```python
from build123d import *

# Parameters (mm, degrees)
SKETCH1_R           = 5
BOSS_EXTRUDE1_DEPTH = 20
SKETCH2_R           = 4
BOSS_EXTRUDE2_DEPTH = 68
FILLET1_R           = 3.4
CHAMFER1_SIZE       = 11.430052303
CHAMFER1_SIZE_2     = 1
SKETCH3_W           = 5
SKETCH3_H           = 5
CUT_EXTRUDE1_DEPTH  = 8
SKETCH4_W           = 5
SKETCH4_H           = 2.702388579
CUT_EXTRUDE2_DEPTH  = 8
SKETCH5_R           = 0.5
BOSS_EXTRUDE3_DEPTH = 5


with BuildPart() as part:
    # Sketch1 → Boss-Extrude1 (new body)
    with BuildSketch(Plane(origin=(0, 0, 0), x_dir=(1, 0, 0), z_dir=(0, 1, 0))):
        with Locations(Location((0, 0, 0), (0, 0, 270))):
            Circle(SKETCH1_R)
    extrude(amount=BOSS_EXTRUDE1_DEPTH)

    # Sketch2 → Boss-Extrude2 (add)
    with BuildSketch(Plane(origin=(0, 20, 0), x_dir=(1, 0, 0), z_dir=(0, 1, 0))):
        with Locations(Location((0, 0, 0), (0, 0, 270))):
            Circle(SKETCH2_R)
    extrude(amount=BOSS_EXTRUDE2_DEPTH)

    # Fillet1
    fillet1_edges = [part.edges().sort_by_distance(p)[0] for p in [
        (0, 88, -4),
    ]]
    fillet(fillet1_edges, radius=FILLET1_R)

    # Chamfer1
    # the kernel refuses this chamfer: 11.430052303, 1 mm, written as the material it adds along each edge
    with BuildSketch(Plane(origin=(0, 20, 0), x_dir=(0, 0, 1), z_dir=(-1, 0, 0))) as chamfer1_piece_1_section:
        Polygon((4, CHAMFER1_SIZE), (4 + CHAMFER1_SIZE_2, 0), (4, 0), align=None)
    chamfer1_piece_1 = revolve(axis=Axis((0, 20, 0), (0, 1, 0)), mode=Mode.PRIVATE)
    chamfer1_piece_1 = chamfer1_piece_1 & Plane(origin=(0, 25.937398898, 0), x_dir=(0, 0, 1), z_dir=(0, -1, 0)) * Cylinder(5, 46, mode=Mode.PRIVATE)
    add(chamfer1_piece_1)

    # Sketch3 → Cut-Extrude1 (cut)
    with BuildSketch(Plane(origin=(0, 0, 0), x_dir=(-1, 0, 0), z_dir=(0, -1, 0))):
        Rectangle(SKETCH3_W, SKETCH3_H)
    extrude(amount=-CUT_EXTRUDE1_DEPTH, mode=Mode.SUBTRACT)

    # Sketch4 → Cut-Extrude2 (cut)
    with BuildSketch(Plane(origin=(0, 0, 0), x_dir=(-1, 0, 0), z_dir=(0, -1, 0))):
        with Locations((0, 3.851194289)):
            Rectangle(SKETCH4_W, SKETCH4_H)
    extrude(amount=-CUT_EXTRUDE2_DEPTH, mode=Mode.SUBTRACT)

    # Sketch5 → Boss-Extrude3 (add)
    with BuildSketch(Plane.ZY.offset(-2.5)):
        with Locations(Location((0, 5.5, 0), (0, 0, 180))):
            Circle(SKETCH5_R)
    extrude(amount=BOSS_EXTRUDE3_DEPTH)


solid = part.part
```
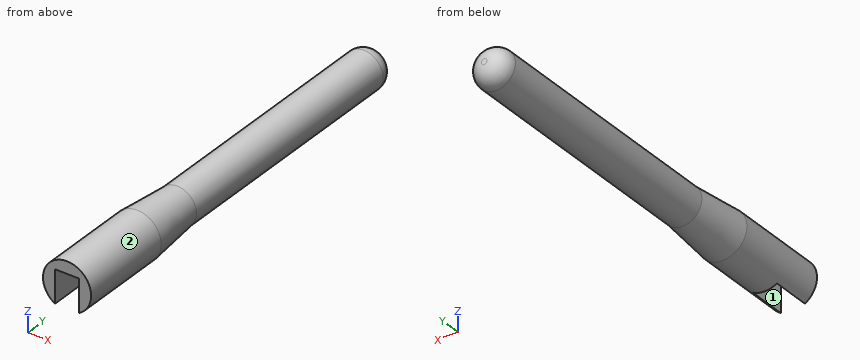
Work out the finished part from the listing and answer in its coordinate system (mm). Face numbers are marked on the shaded views. Coordinates: 2 decimals unless noted, no trailing zeros. Order: outer loops, then holes, each group sorted by start corner. A loop starts at its lowest first (then second) coordinate and runs counter-clockwise, first axis right, second up. Notation, with made-up numbers: M -37.75,2.25 L -31.75,2.25 A23 cw -31.75,36.25 Z; hole C 45,28.25 d8. An arc over 180 degrees is marked long. Use CSV: the item, a comma, the result in double quotes.
1) Determine the mould class of the marked faces 1 and 2 for opening direction X: released by +X, released by -X, zero draft, split by the parting line, or undercut.
Worked out:
face 1,"undercut"
face 2,"split by the parting line"
2) Flat-ended cylindrical pins translate along their axes: pin 1 Ø3.5 at (y, z) = (4, -2.5) entering from +X; pin 2 Ø3 at (y, z) = (45.5, -1.5) entering from -X; pin 3 Ø1.5 at (x, y) = (0.5, 4) entering from -Z. Find the tip coordinate at first contact, or state that the pin passes through.
Worked out:
pin 1,"stops at x = 4.94"
pin 2,"stops at x = -4"
pin 3,"stops at z = 2.5"
3) Section B-B on y = 10 is taken. Write down the section's boundary in (x, z).
Worked out:
outline,"C 0,0 d10"
4) Section A-A on y = 66.5 is taken. Write down the section's boundary in (x, z), plus the area to 3 significant figures.
Worked out:
outline,"C 0,0 d8"
area,"50.3 mm^2"
5) Consider line 1 (Z direction, x = -2.75, y = 21.5); line 2 (Y direction, x = -2, z = 0); line 3 (X direction, y = 58, z = -1.5). Determine where each line is inside the solid, lowest interval first. Write a range as [from, to].
Worked out:
line 1,"z = [-4.02, 4.02]"
line 2,"y = [5, 6], [8, 87.7]"
line 3,"x = [-3.71, 3.71]"
